from build123d import *

# Parameters (mm, degrees)
F0_W       = 99
F0_H       = 150
F1_DEPTH   = 1
F1_FACE1_W = 99
F1_FACE1_H = 150
F2_R       = 5.8629456908
F3_DEPTH   = 1
F4_DEPTH   = 25
F6_DEPTH   = 25


with BuildPart() as f1:
    # F0 (on Front) → F1 (new body)
    with BuildSketch(Plane.XZ):
        Rectangle(F0_W, F0_H)
    extrude(amount=F1_DEPTH)

    # F1_face1 (on face) + F2 (on face) → F3 (join)
    with BuildSketch(Plane.XZ.offset(1)):
        Rectangle(F1_FACE1_W, F1_FACE1_H)
    with BuildSketch(Plane(origin=(0, 0, 0), x_dir=(-1, 0, 0), z_dir=(0, 1, 0))):
        with Locations((6.8623106927, -62.4270327389)):
            Circle(F2_R)
    extrude(amount=F3_DEPTH, dir=(0, -1, 0))

    # F2 (on face) → F4 (cut)
    with BuildSketch(Plane(origin=(0, 0, 0), x_dir=(-1, 0, 0), z_dir=(0, 1, 0))):
        with Locations((6.8623106927, -62.4270327389)):
            Circle(F2_R)
    extrude(amount=-F4_DEPTH, mode=Mode.SUBTRACT)

    # F5 (on face) → F6 (cut)
    with BuildSketch(Plane(origin=(0, 0, 0), x_dir=(-1, 0, 0), z_dir=(0, 1, 0))):
        Polygon((-49.5, -75), (-19.9534265946, -75), (-19.9534265946, 31), (-23.702466874, 36.5829747168), (-46.8139478722, 71), (-49.5, 75), align=None)
        Polygon((26.5, 31), (26.5, -75), (49.5, -75), (49.5, 75), (47.6940077596, 75), (45.7672797814, 71), (29.1892183971, 36.5829747168), align=None)
    extrude(amount=-F6_DEPTH, mode=Mode.SUBTRACT)


solid = f1.part
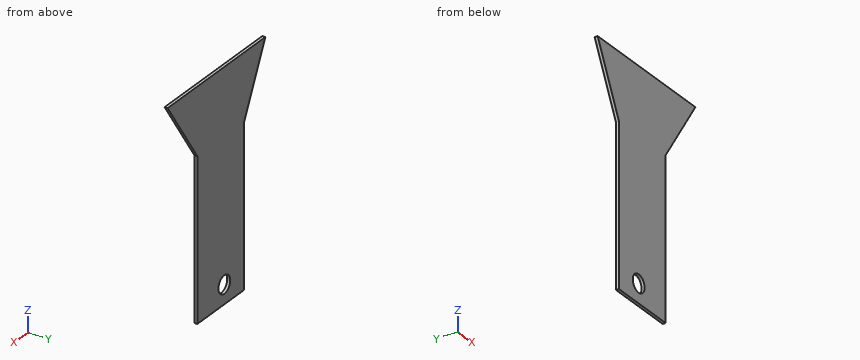
Could you check a few things on this model? Use its own coordinates, in mm. Give positions to 0.01 mm unless a question says otherwise; leave off trailing zeros. Loops run counter-clockwise (first coordinate to the right, second up) from the corner with the lowest first, then second, coordinate; pieces in that order, holes last. Notation, with made-up numbers: M 38.5,61.25 L 59.5,61.25 A28 ccw 59.5,92.25 Z; hole C 67,-11.5 d3. An arc over 180 degrees is marked long. Answer as a JSON object with one key per item and string values.
Q1. If I drill on probe 1 along X at (y, z) = (-1.2, 28.5); probe 2 along Z at (x, y) = (-2, -1.05); probe 3 along Z at (x, y) = (-5.5, -1.8), over which ranges is the centre line in solid material (lowest first)? Write a range as [from, to].
Values found:
{"probe 1": "x = [-26.5, 19.95]", "probe 2": "z = [-75, -65.7], [-59.15, 75]", "probe 3": "z = [-75, -68.13], [-56.72, 75]"}
Q2. Suppose I cut it at D-D, the plane x = -38.5. List the corners of the cut face in (y, z) for me.
Values found:
{"outline": "M -2,55.91 L 0,55.91 L 0,75 L -2,75 Z"}
Q3. Suppose I cut it at A-A, the plane x = -4. List the corners of the cut face in (y, z) for me, plus the area to 3 significant figures.
Values found:
{"outline": "M -2,-75 L 0,-75 L 0,-67.54 L -2,-67.54 Z; M -2,-57.31 L 0,-57.31 L 0,75 L -2,75 Z", "area": "280 mm²"}
Q4. For P1, Ø1, axis at y = -1.5, z = 51.5, coming from the -X side; P2, Ø0.6, axis at y = -0.5, z = -38, coming from the +X side; P3, Ø7, axis at x = -6.86, z = -62.43, coming from the -Y side, each with a flat end and sliding along its axis, tell me the tip position at first contact or that it passes through.
Values found:
{"P1": "stops at x = -36.62", "P2": "stops at x = 19.95", "P3": "passes through"}
Q5. Suppose I cut it at B-B, the plane y = -1.05. List the corners of the cut face in (x, z) for me, plus the area to 3 significant figures.
Values found:
{"outline": "M -47.69,75 L -26.5,31 L -26.5,-75 L 19.95,-75 L 19.95,31 L 49.5,75 Z; hole C -6.86,-62.43 d11.73", "area": "7,980 mm²"}
Q6. Suppose I cut it at C-C, the plane z = -3. List the corners of the cut face in (x, y) for me, plus the area to 3 significant figures.
Values found:
{"outline": "M -26.5,-2 L 19.95,-2 L 19.95,0 L -26.5,0 Z", "area": "92.9 mm²"}
